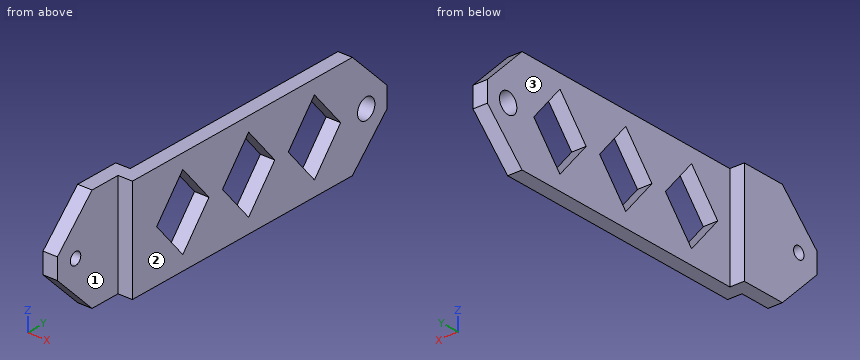
```python
from build123d import *

# Parameters (mm, degrees)
F1_DEPTH = 50
F2_R     = 3
F2_R_2   = 5
F3_DEPTH = 25
F5_DEPTH = 25
F6_SIZE2 = 20
F6_SIZE  = 20


with BuildPart() as f1:
    # F0 (on Top) → F1 (new body)
    with BuildSketch(Plane.XY):
        Polygon((-14, 7), (-14, -35), (-7, -35), (-7, 0), (0, 0), (0, 147), (-7, 147), (-7, 7), align=None)
    extrude(amount=F1_DEPTH)

    # F2 (on Right) → F3 (cut)
    with BuildSketch(Plane.YZ):
        with Locations((-24.5, 25)):
            Circle(F2_R)
        with Locations((135, 25)):
            Circle(F2_R_2)
    extrude(amount=-F3_DEPTH, mode=Mode.SUBTRACT)

    # F4 (on face) → F5 (cut)
    with BuildSketch(Plane(origin=(-7, 0, 0), x_dir=(0, -1, 0), z_dir=(-1, 0, 0))):
        Polygon((-89.999746, 25.19642), (-105.10354, 43.19642), (-120.207333, 25.19642), (-105.10354, 7.19642), align=None)
        Polygon((-51.999873, 25.09821), (-67.103666, 43.09821), (-82.20746, 25.09821), (-67.103666, 7.09821), align=None)
        Polygon((-44.207587, 25), (-29.103793, 7), (-14, 25), (-29.103793, 43), align=None)
    extrude(amount=-F5_DEPTH, mode=Mode.SUBTRACT)

    # F6
    f6_edges = [f1.edges().sort_by_distance(p)[0] for p in [
        (-3.5, 147, 50),
        (-3.5, 147, 0),
        (-10.5, -35, 50),
        (-10.5, -35, 0),
    ]]
    chamfer(f6_edges, length=F6_SIZE, length2=F6_SIZE2)


solid = f1.part
```
Could you check a few things on this model? Use its own coordinates, in mm. Face numbers are marked on the shaded views. A direction names the side the tool comes from. Give positions to 0.01 mm unless a question says otherwise; leave off trailing zeros. Order: outer loops, then holes, each group sorted by start corner. A loop starts at its lowest first (then second) coordinate and runs counter-clockwise, first axis right, second up.
Q1. Suppose I cut it at D-D, the plane y = -24.5. Write out the boundary of the cut face in (x, z), and give its area (3 significant figures).
Q2. Suppose I cut it at B-B, the plane x = -5. Write out the boundary of the cut face in (y, z).
Q3. Suppose I cut it at A-A, the plane y = 135. Write out the boundary of the cut face in (x, z).
Q4. Suppose I cut it at C-C, the plane z = 38.5. Write out the boundary of the cut face in (x, y), and give its area (3 significant figures).
Q5. I'm going to push flat-ended pins straight in: P1, Ø3.5, axis at x = -11.5, z = 28, coming from the +Y side; P2, Ø5, axis at y = 86, z = 36.5, coming from the -X side; P3, Ø5.5, axis at x = -4, z = 14, coming from the -Y side; P4, Ø11.5, axis at y = 135, z = 25, coming from the +X side. Where does each tip first touch, or does it pass through?
Q6. If I drill on line 1 along Y through (x, z) = (-4.5, 22); line 2 along X through (y, z) = (39, 37.5); line 3 along Y through (x, z) = (-4, 42.5), over which ranges is the centre line in solid material (lowest first)?
Q7. For the marked faces 1, 2 and 3, which set-ups out of +Z, -Z, +X, -X, +Y, -Y let a thin tool reach every point of the face, with its end or its side?
Solution:
1. outline: (-14, 9.5) - (-7, 9.5) - (-7, 22) - (-14, 22) - close; (-14, 28) - (-7, 28) - (-7, 40.5) - (-14, 40.5) - close
1. area: 175 mm2
2. outline: (0, 0) - (127, 0) - (147, 20) - (147, 30) - (127, 50) - (0, 50) - close; hole (14, 25) - (29.1, 7) - (44.21, 25) - (29.1, 43) - close; hole (52, 25.1) - (67.1, 7.1) - (82.21, 25.1) - (67.1, 43.1) - close; hole (90, 25.2) - (105.1, 7.2) - (120.21, 25.2) - (105.1, 43.2) - close; hole circle Ø10 at (135, 25)
3. outline: (-7, 8) - (0, 8) - (0, 20) - (-7, 20) - close; (-7, 30) - (0, 30) - (0, 42) - (-7, 42) - close
4. outline: (-14, -26.5) - (-7, -26.5) - (-7, 0) - (0, 0) - (0, 25.33) - (-7, 25.33) - (-7, 7) - (-14, 7) - close; (-7, 32.88) - (0, 32.88) - (0, 63.25) - (-7, 63.25) - close; (-7, 70.96) - (0, 70.96) - (0, 101.16) - (-7, 101.16) - close; (-7, 109.04) - (0, 109.04) - (0, 138.5) - (-7, 138.5) - close
4. area: 1,040 mm2
5. P1: stops at y = 7
5. P2: stops at x = -7
5. P3: stops at y = 0
5. P4: stops at x = 0
6. line 1: y = 0 to 16.52, 41.69 to 54.6, 79.61 to 92.68, 117.53 to 131, 139 to 147
6. line 2: x = -7 to 0
6. line 3: y = 0 to 28.68, 29.52 to 66.6, 67.61 to 104.52, 105.69 to 134.5
7. face 1: +Z, -Z, +X, -Y
7. face 2: +Z, -Z, +X, +Y, -Y
7. face 3: +Z, -Z, -X, +Y
